Check sheet for the modelled part. Datum: model origin and axes. Units: mm. A direction names the side the tool comes from. Coordinates: 2 decimals unless noted, no trailing zeros. Loops run counter-clockwise (first coordinate to the right, second up) from the corner with the lowest first, then second, coordinate; pieces in that order, holes last. Notation, with made-up numbers: M 74.25,61 L 126.25,61 A19 cw 126.25,72 Z; hole C 56,80.5 d3. An arc over 180 degrees is marked long. Answer in a Markdown table with one row per item. Add a question column.
```python
from build123d import *

# Parameters (mm, degrees)
ESQUISSE1_W             = 30
ESQUISSE1_H             = 50
ESQUISSE1_R             = 10
BOSS_EXTRU_1_DEPTH      = 50
ESQUISSE3_R             = 29.154759474
BOSS_EXTRU_2_DEPTH      = 66
ESQUISSE4_R             = 20
ENL_V_MAT_EXTRU_1_DEPTH = 25


with BuildPart() as part:
    # Esquisse1 → Boss.-Extru.1 (new body)
    with BuildSketch(Plane.XY):
        with Locations((-293.597239891, -30)):
            Rectangle(ESQUISSE1_W, ESQUISSE1_H)
        with Locations((-293.597239891, -40)):
            Circle(ESQUISSE1_R, mode=Mode.SUBTRACT)
    extrude(amount=BOSS_EXTRU_1_DEPTH)

    # Esquisse3 → Boss.-Extru.2 (add)
    with BuildSketch(Plane(origin=(0, -5, 0), x_dir=(1, 0, 0), z_dir=(0, 1, 0))):
        with Locations(Location((-293.597239891, -25, 0), (0, 0, 59.036243468))):
            Circle(ESQUISSE3_R)
    extrude(amount=BOSS_EXTRU_2_DEPTH)

    # Esquisse4 → Enlèv. mat.-Extru.1 (cut)
    with BuildSketch(Plane(origin=(0, 61, 0), x_dir=(1, 0, 0), z_dir=(0, 1, 0))):
        with Locations(Location((-293.597239891, -25, 0), (0, 0, 270))):
            Circle(ESQUISSE4_R)
    extrude(amount=-ENL_V_MAT_EXTRU_1_DEPTH, mode=Mode.SUBTRACT)


solid = part.part
```
Q1. Thickness scan on L1, parallel to Y at x = -293, z = 18; L2, parallel to X at y = 48, z = 25; L3, parallel to X at y = -39.5, z = 32. Record the ranges inside material, lowest first.
Q2. Cross-section at D-D (y = 34). Record the cut outline in (x, z), plus the area to 3 significant figures.
Q3. Go/stop test with flat-tipped pins: pin 1 (2 mm diameter, centred on y = 23.5, z = 40.5, fed in from +X); pin 2 (8 mm diameter, centred on x = -277, y = 22.5, fed in from -Z); pin 3 (4 mm diameter, centred on x = -313, z = 24, fed in from -Y). Record where each tip stops, or that it passes through.
Q4. Cross-section at C-C (z = 19.5). Record the cut outline in (x, y), plus the area to 3 significant figures.
Q5. Access from +Z, -Z, +X, -X, +Y, -Y to the whole of each face (thin tool, end or side, straight path). Record for faces 1 (the face through (-294, -5, 52)), 2 (the face through (-316, -5, 27)), 3 (the face through (-272, -5, 24)), 4 (the face through (-293, -5, -2)).
Q6. Cross-section at A-A (x = -298.5). Record the cut outline in (y, z), plus the area to 3 significant figures.
Q7. Cross-section at B-B (y = -40). Record the cut outline in (x, z).
Q8. Mould release check, pull along X, two halves, no side actions. Record for faces 5 (the face through (-293, 36, 25)), 6 (the face through (-278.597, -30, 25)), 7 (the face through (-281, 61, 41)), 8 (the face through (-308.597, -30, 25)): released by +X, released by -X, zero draft, split by the parting line, or undercut.
Answer key:
| question | item | result |
|---|---|---|
| 1 | L1 | -55 to -49.98, -30.02 to 36 |
| 1 | L2 | -322.75 to -313.6, -273.6 to -264.44 |
| 1 | L3 | -308.6 to -303.58, -283.61 to -278.6 |
| 2 | outline | C -293.6,25 d58.31 |
| 2 | area | 2,670 mm^2 |
| 3 | pin 1 | x = -268.3 |
| 3 | pin 2 | z = -1.29 |
| 3 | pin 3 | y = -5 |
| 4 | outline | M -322.23,-5 L -308.6,-5 L -308.6,-55 L -278.6,-55 L -278.6,-5 L -264.97,-5 L -264.97,61 L -274.37,61 L -274.37,36 L -312.83,36 L -312.83,61 L -322.23,61 Z; hole C -293.6,-40 d20 |
| 4 | area | 4,000 mm^2 |
| 5 | face 1 | +Z, +X, -X, -Y |
| 5 | face 2 | +Z, -Z, -X, -Y |
| 5 | face 3 | +Z, -Z, +X, -Y |
| 5 | face 4 | -Z, +X, -X, -Y |
| 6 | outline | M -55,0 L -48.72,0 L -48.72,50 L -55,50 Z; M -31.28,0 L -5,0 L -5,-3.74 L 61,-3.74 L 61,5.61 L 36,5.61 L 36,44.39 L 61,44.39 L 61,53.74 L -5,53.74 L -5,50 L -31.28,50 Z |
| 6 | area | 4,450 mm^2 |
| 7 | outline | M -308.6,0 L -303.6,0 L -303.6,50 L -308.6,50 Z; M -283.6,0 L -278.6,0 L -278.6,50 L -283.6,50 Z |
| 8 | face 5 | undercut |
| 8 | face 6 | released by +X |
| 8 | face 7 | zero draft |
| 8 | face 8 | released by -X |
